```python
from build123d import *

# Parameters (mm, degrees)
BOSS_EXTRUDE1_DEPTH             = 1.5
BOSS_EXTRUDE2_DEPTH             = 1.5
BOSS_EXTRUDE3_DEPTH             = 1.5
CUT_EXTRUDE1_START              = -4
SKETCH2_R                       = 2.25
CUT_EXTRUDE1_DEPTH              = 5
CIRPATTERN1_COUNT               = 3
CIRPATTERN1_ANGLE               = 60
CIRPATTERN1_THE_OTHER_WAY_COUNT = 3
CIRPATTERN1_THE_OTHER_WAY_ANGLE = 60
CUT_EXTRUDE2_START              = -4
SKETCH6_R                       = 2.25
CUT_EXTRUDE2_DEPTH              = 5
LPATTERN1_COUNT                 = 2
LPATTERN1_PITCH                 = 15
LPATTERN1_COUNT_DIR2            = 2
LPATTERN1_PITCH_DIR2            = 10
LPATTERN2_COUNT                 = 2
LPATTERN2_PITCH                 = 15
LPATTERN2_COUNT_DIR2            = 2
LPATTERN2_PITCH_DIR2            = 10


with BuildPart() as part:
    # Sketch1 → Boss-Extrude1 (new body, symmetric)
    with BuildSketch(Plane(origin=(0, 0, 0), x_dir=(1, 0, 0), z_dir=(0, 1, 0))):
        with BuildLine():
            Line((0, 33), (0, 43))
            ThreePointArc((0, 43), (41.53481053, 11.129218939), (21.5, -37.239092363))
            Line((21.5, -37.239092363), (16.5, -28.578838325))
            ThreePointArc((16.5, -28.578838325), (31.875552268, 8.541028488), (0, 33))
        make_face()
    extrude(amount=BOSS_EXTRUDE1_DEPTH, both=True)

    # Sketch4 → Boss-Extrude2 (add, symmetric)
    with BuildSketch(Plane(origin=(0, 0, 0), x_dir=(1, 0, 0), z_dir=(0, 1, 0))):
        Polygon((68.871738323, 44.336031175), (25.40507614, 32.689174146), (38.346028395, -15.607117169), (81.812690578, -3.960260139), align=None)
    extrude(amount=BOSS_EXTRUDE2_DEPTH, both=True)

    # Sketch5 → Boss-Extrude3 (add, symmetric)
    with BuildSketch(Plane(origin=(0, 0, 0), x_dir=(1, 0, 0), z_dir=(0, 1, 0))):
        Polygon((0, 43), (48.097432179, 38.769572621), (27.323126035, 33.203114066), align=None)
        Polygon((61.038384434, -9.526718694), (40.26407829, -15.093177248), (21.5, -37.239092363), align=None)
    extrude(amount=BOSS_EXTRUDE3_DEPTH, both=True)

    # Sketch2 → Cut-Extrude1 (cut)
    with BuildSketch(Plane(origin=(0, 1.5, 0), x_dir=(1, 0, 0), z_dir=(0, 1, 0)).offset(CUT_EXTRUDE1_START)):
        with Locations((36.757261811, 9.638656763)):
            Circle(SKETCH2_R)
    cut_extrude1 = extrude(amount=CUT_EXTRUDE1_DEPTH, mode=Mode.SUBTRACT)

    # CirPattern1: Cut-Extrude1 ×3 about axis
    cirpattern1_axis = Axis((0, 0, 0), (0, -1, 0))
    for i in range(1, CIRPATTERN1_COUNT):
        add(cut_extrude1.rotate(cirpattern1_axis, i * CIRPATTERN1_ANGLE / (CIRPATTERN1_COUNT - 1)), mode=Mode.SUBTRACT)

    # CirPattern1 the other way: Cut-Extrude1 ×3 about axis
    cirpattern1_the_other_way_axis = Axis((0, 0, 0), (0, 1, 0))
    for i in range(1, CIRPATTERN1_THE_OTHER_WAY_COUNT):
        add(cut_extrude1.rotate(cirpattern1_the_other_way_axis, i * CIRPATTERN1_THE_OTHER_WAY_ANGLE / (CIRPATTERN1_THE_OTHER_WAY_COUNT - 1)), mode=Mode.SUBTRACT)

    # Sketch6 → Cut-Extrude2 (cut)
    with BuildSketch(Plane(origin=(0, 1.5, 0), x_dir=(1, 0, 0), z_dir=(0, 1, 0)).offset(CUT_EXTRUDE2_START)):
        with Locations((70.512585319, 18.893790292)):
            Circle(SKETCH6_R)
    cut_extrude2 = extrude(amount=CUT_EXTRUDE2_DEPTH, mode=Mode.SUBTRACT)

    # LPattern1: Cut-Extrude2 2 × 2
    with Locations(*[Vector(-0.258819045, 0, -0.965925826) * (i * LPATTERN1_PITCH) + Vector(-0.965925826, 0, 0.258819045) * (j * LPATTERN1_PITCH_DIR2) for i in range(LPATTERN1_COUNT) for j in range(LPATTERN1_COUNT_DIR2) if (i, j) != (0, 0)]):
        add(cut_extrude2, mode=Mode.SUBTRACT)

    # LPattern2: Cut-Extrude2 2 × 2
    with Locations(*[Vector(0.258819045, 0, 0.965925826) * (i * LPATTERN2_PITCH) + Vector(-0.965925826, 0, 0.258819045) * (j * LPATTERN2_PITCH_DIR2) for i in range(LPATTERN2_COUNT) for j in range(LPATTERN2_COUNT_DIR2) if (i, j) != (0, 0)]):
        add(cut_extrude2, mode=Mode.SUBTRACT)


solid = part.part
```
Could you check a few things on this model? Use its own coordinates, in mm. A direction names the side the tool comes from. Round coordinates to 2 decimals unless told otherwise and drop trailing zeros. Loops run counter-clockwise (first coordinate to the right, second up) from the corner with the lowest first, then second, coordinate; pieces in that order, holes last.
Q1. Thinking about a two-plate mould opening in Z: for faces 3 (the cylindrical face through (59.068, -0.021, -14.937)), 4 (the cylindrical face through (63.08, -0.02, -3.34)), 5 (the flat face through (49, -1.5, -13)), 6 (the cylindrical face through (24.7, 0, 35.2)), which applies, pulls with the +Z half, pulls with the -Z half, needs draft (parallel to the pull), parting line crosses it, or undercut?
Q2. I want a section at C-C (y = -0.3). Give the number of separate pieces and of enclosed holes in the cut face, and give its area (3 significant figures).
Q3. On a 3-axis mill with a long thin cutter (end or side, diameter ignored), from which of +Z, -Z, +X, -X, +Y, -Y can I reach the whole of each face in a straight line? I mean faces 1 (the cylindrical face through (3.71, 0.02, -42.84)), 2 (the flat face through (19.035, 0.021, 32.97)). Say none if no direction works.
Q4. Please list where these lines run through material, in increasing order: L1, parallel to Z at x = 65, y = -0.7; L2, parallel to X at y = 0.8, z = -30; L3, parallel to X at y = 0.8, z = -33.5.
Q5. I want a section at A-A (x = 70.5). Write out the boundary of the cut face in (y, z).
Q6. I want a section at D-D (x = 43). Write out the boundary of the cut face in (y, z), and give its area (3 significant figures).
Q7. I want a section at B-B (z = 26). Write out the boundary of the cut face in (x, y), and give its area (3 significant figures).
Answer below:
1. face 3: undercut
1. face 4: undercut
1. face 5: needs draft
1. face 6: pulls with the +Z half
2. separate pieces: 1
2. enclosed holes: 11
2. area: 2,960 mm2
3. face 1: -Z, +Y, -Y
3. face 2: +Z, -X, +Y, -Y
4. L1: z = -43.3 to -34.93, -31.83 to -4.05, 0.42 to 8.47
4. L2: x = 13.75 to 54.87, 59.08 to 72.71
4. L3: x = 0 to 64.38, 68.88 to 71.78
5. outline: (-1.5, -38.26) - (1.5, -38.26) - (1.5, -21.14) - (-1.5, -21.14) - close; (-1.5, -16.64) - (1.5, -16.64) - (1.5, 6.99) - (-1.5, 6.99) - close
6. outline: (-1.5, -39.22) - (1.5, -39.22) - (1.5, 22.17) - (-1.5, 22.17) - close
6. area: 184 mm2
7. outline: (20.32, -1.5) - (24.72, -1.5) - (24.72, 1.5) - (20.32, 1.5) - close; (28.73, -1.5) - (37.54, -1.5) - (37.54, 1.5) - (28.73, 1.5) - close
7. area: 39.6 mm2
